Check sheet for the modelled part. Datum: model origin and axes. Units: mm. A direction names the side the tool comes from. Give positions to 0.01 mm unless a question says otherwise; leave off trailing zeros. Loops run counter-clockwise (first coordinate to the right, second up) from the corner with the lowest first, then second, coordinate; pieces in that order, holes last. Notation, with made-up numbers: (53, 46) - (84, 46) arc R22 ccw to (84, 56) - close; hole circle Ø11 at (9.5, 12.25). An arc over 180 degrees is marked (long way). Answer in a Markdown table with one row per item. Add a question column.
(1) Set-up check for faces 1 (the face through (24.54, 186.92, 75.13)), 2 (the face through (23.541, 185.664, 75.133)): record each of +Z, -Z, +X, -X, +Y, -Y from which the full face is reachable in a straight line by a thin tool's end or side.
(2) Sectioned sample at D-D on x = -1. Enter the section's corners in (y, z).
(3) Sectioned sample at C-C on y = 158. Enter the section's corners in (x, z).
(4) Go/stop test with flat-tipped pins: P1, Ø2, axis at y = 188.5, z = 96.5, coming from the +X side; P2, Ø3, axis at x = 10.5, z = 66, coming from the +Y side; P3, Ø1.5, axis at y = 158.5, z = 51.5, coming from the +X side. Record where each tip stops, or that it passes through.
(5) Sectioned sample at A-A on y = 182. Enter the section's corners in (x, z).
(6) Thickness scan on L1, parallel to X at y = 167.5, z = 93; L2, parallel to X at y = 151, z = 101; L3, parallel to Y at x = 27, z = 72.5. Record the ranges inside material, lowest first.
from build123d import *

# Parameters (mm, degrees)
BOSS_EXTRUDE2_DEPTH = 152.4


with BuildPart() as part:
    # Sketch1 → Boss-Extrude2 (new body)
    with BuildSketch(Plane.XY):
        with BuildLine():
            Line((37.717239544, 147.658964649), (35.965487423, 153.043027332))
            Line((35.965487423, 153.043027332), (33.550115758, 152.257164929))
            Line((33.550115758, 152.257164929), (30.406666146, 161.918651592))
            Line((30.406666146, 161.918651592), (32.822037812, 162.704513995))
            Line((32.822037812, 162.704513995), (32.036175409, 165.119885661))
            Line((32.036175409, 165.119885661), (27.627587493, 178.669812847))
            ThreePointArc((27.627587493, 178.669812847), (23.462294361, 185.748899875), (16.703713988, 190.41631151))
            ThreePointArc((16.703713988, 190.41631151), (0, 193.690277018), (-16.703713988, 190.41631151))
            ThreePointArc((-16.703713988, 190.41631151), (-23.462294361, 185.748899875), (-27.627587493, 178.669812847))
            Line((-27.627587493, 178.669812847), (-32.036175409, 165.119885661))
            Line((-32.036175409, 165.119885661), (-32.822037812, 162.704513995))
            Line((-32.822037812, 162.704513995), (-30.406666146, 161.918651592))
            Line((-30.406666146, 161.918651592), (-33.550115758, 152.257164929))
            Line((-33.550115758, 152.257164929), (-35.965487423, 153.043027332))
            Line((-35.965487423, 153.043027332), (-37.717239544, 147.658964649))
            ThreePointArc((-37.717239544, 147.658964649), (-38.630482432, 147.422677452), (-39.542245278, 147.180742077))
            Line((-39.542245278, 147.180742077), (-29.137194784, 179.160976849))
            ThreePointArc((-29.137194784, 179.160976849), (-24.624793891, 186.829987796), (-17.302998471, 191.886350359))
            ThreePointArc((-17.302998471, 191.886350359), (0, 195.277776974), (17.302998471, 191.886350359))
            ThreePointArc((17.302998471, 191.886350359), (24.624793891, 186.829987796), (29.137194784, 179.160976849))
            Line((29.137194784, 179.160976849), (39.542245278, 147.180742077))
            ThreePointArc((39.542245278, 147.180742077), (38.630482432, 147.422677452), (37.717239544, 147.658964649))
        make_face()
    extrude(amount=BOSS_EXTRUDE2_DEPTH)


solid = part.part
Reply:
| question | item | result |
|---|---|---|
| 1 | face 1 | +Z, -Z, +X, +Y |
| 1 | face 2 | +Z, -Z, -Y |
| 2 | outline | (193.68, 0) - (195.27, 0) - (195.27, 152.4) - (193.68, 152.4) - close |
| 3 | outline | (-36.02, 0) - (-31.68, 0) - (-31.68, 152.4) - (-36.02, 152.4) - close; (31.68, 0) - (36.02, 0) - (36.02, 152.4) - (31.68, 152.4) - close |
| 4 | P1 | x = 23.97 |
| 4 | P2 | y = 194.39 |
| 4 | P3 | x = 36.1 |
| 5 | outline | (-27.97, 0) - (-26.18, 0) - (-26.18, 152.4) - (-27.97, 152.4) - close; (26.18, 0) - (27.97, 0) - (27.97, 152.4) - (26.18, 152.4) - close |
| 6 | L1 | -32.93 to -31.26, 31.26 to 32.93 |
| 6 | L2 | -38.3 to -36.63, 36.63 to 38.3 |
| 6 | L3 | 180.33 to 183.73 |
